Check sheet for the modelled part. Datum: model origin and axes. Units: mm. Round coordinates to 2 decimals unless told otherwise and drop trailing zeros. Loops run counter-clockwise (first coordinate to the right, second up) from the corner with the lowest first, then second, coordinate; pieces in that order, holes last. Notation, with made-up numbers: (81.5, 38.25) - (135.5, 38.25) arc R9 cw to (135.5, 51.25) - close; hole circle Ø11 at (80, -4.75). An arc over 180 degrees is marked (long way). Answer in a Markdown table with one row per item. Add a question column.
(1) Thickness scan on line 1 along Y through (x, z) = (10, 2.3); line 2 along X through (y, z) = (100, 3.95); line 3 along Y through (x, z) = (18.5, 2.3). Record the ranges inside material, lowest first.
(2) Cross-section at A-A on z = 2.6. Count the separate pieces of the cut face and the enclosed holes in it, then the cut area to 3 significant figures.
(3) Cross-section at C-C on x = 17. Enter the section's corners in (y, z).
(4) Mould release check, pull along X, two halves, no side actions. Record for faces 1 (the cylindrical face through (2.85, 3.01, 2.54)), 2 (the cylindrical face through (16.99, 197.15, 2.54)), 3 (the cylindrical face through (10.89, 41.39, 2.46)): +X half, -X half, draft (parallel to the pull), parting line (faces both ways), or undercut.
(5) Gauge pin test, flat ends, axial feed: pin 1 (2 mm diameter, centred on x = 2, z = 3, fed in from -Y); pin 2 (1 mm diameter, centred on x = 9, z = 3.5, fed in from -Y); pin 3 (1 mm diameter, centred on x = 17, z = 0.5, fed in from +Y); pin 4 (3 mm diameter, centred on x = 10, y = 40, fed in from -Z). Record the tip position at first contact, or that the pin passes through.
(6) Cross-section at B-B on y = 40. Enter the section's corners in (x, z).
(7) Cross-section at D-D on x = 3.25. Enter the section's corners in (y, z).
from build123d import *

# Parameters (mm, degrees)
SKETCH1_W           = 20
SKETCH1_H           = 200
SKETCH1_R           = 1.65
BOSS_EXTRUDE1_DEPTH = 5
FILLET1_R           = 10


with BuildPart() as part:
    # Sketch1 → Boss-Extrude1 (new body)
    with BuildSketch(Plane.XY):
        with Locations((10, 100)):
            Rectangle(SKETCH1_W, SKETCH1_H)
        with Locations((10, 160)):
            Circle(SKETCH1_R, mode=Mode.SUBTRACT)
        with Locations((10, 100)):
            Circle(SKETCH1_R, mode=Mode.SUBTRACT)
        with Locations((10, 40)):
            Circle(SKETCH1_R, mode=Mode.SUBTRACT)
    extrude(amount=BOSS_EXTRUDE1_DEPTH)

    # Fillet1
    fillet1_edges = [part.edges().sort_by_distance(p)[0] for p in [
        (0, 0, 2.5),
        (20, 0, 2.5),
        (20, 200, 2.5),
        (0, 200, 2.5),
    ]]
    fillet(fillet1_edges, radius=FILLET1_R - 0.0001)  # a hair under: the kernel refuses the full size


solid = part.part
Answers:
| question | item | result |
|---|---|---|
| 1 | line 1 | y = 0 to 38.35, 41.65 to 98.35, 101.65 to 158.35, 161.65 to 200 |
| 1 | line 2 | x = 0 to 8.35, 11.65 to 20 |
| 1 | line 3 | y = 4.73 to 195.27 |
| 2 | separate pieces | 1 |
| 2 | enclosed holes | 3 |
| 2 | area | 3,890 mm^2 |
| 3 | outline | (2.86, 0) - (197.14, 0) - (197.14, 5) - (2.86, 5) - close |
| 4 | face 1 | -X half |
| 4 | face 2 | +X half |
| 4 | face 3 | undercut |
| 5 | pin 1 | stops at y = 2.86 |
| 5 | pin 2 | stops at y = 0.01 |
| 5 | pin 3 | stops at y = 197.6 |
| 5 | pin 4 | passes through |
| 6 | outline | (0, 0) - (8.35, 0) - (8.35, 5) - (0, 5) - close; (11.65, 0) - (20, 0) - (20, 5) - (11.65, 5) - close |
| 7 | outline | (2.62, 0) - (197.38, 0) - (197.38, 5) - (2.62, 5) - close |
